Can you work these out from the model? Positions are in its coordinate system, mm. A direction names the side the tool comes from. Give positions to 0.01 mm unless a question says otherwise; leave off trailing zeros. Order: outer loops, then holes, each group sorted by start corner. A loop starts at its lowest first (then second) coordinate and runs counter-clockwise, first axis right, second up.
Item 1: I want a section at C-C, the plane y = 112. Write out the boundary of the cut face in (x, z).
Item 2: Which directions (+Z, -Z, +X, -X, +Y, -Y) give clear straight access to the entire face, cutting with the end or side of a thin tool? Please do faces 4 (the flat face through (-1, 291, -4.034)), 5 (the flat face through (-24.772, 291, 9)).
Item 3: I want a section at A-A, the plane y = 565.15. Write out the boundary of the cut face in (x, z).
Item 4: I'm going to push a flat-ended pin straight in: pin 1 Ø6 at (x, z) = (17, 10) entering from +Y. Where does the tip first touch, or does it pass through?
Item 5: If we mould it in two halves opening along X, with no side actions, what happens to faces 1 (the flat face through (24.504, 291, 9)), 2 (the flat face through (-26.296, 291, 9)), 3 (the flat face through (-1, 291, -2.51))? For each: +X half, -X half, draft (parallel to the pull), parting line (faces both ways), or undercut.
Item 6: I want a section at B-B, the plane z = 11. Write out the boundary of the cut face in (x, y).
Item 7: I want a section at D-D, the plane x = -1. Write out the boundary of the cut face in (y, z).
Item 8: If I drill on line 1 along Z through (x, y) = (-17, 196.5); line 2 along X through (y, z) = (402.5, 8); line 3 along X through (y, z) = (565.15, -3.4), over which ranges is the centre line in solid material (lowest first)?
```python
from build123d import *

# Parameters (mm, degrees)
SKETCH1_W           = 50.8
SKETCH1_H           = 25.4
SKETCH1_W_2         = 47.752
SKETCH1_H_2         = 22.352
BOSS_EXTRUDE2_DEPTH = 590.55
SKETCH2_R           = 7.9375
CUT_EXTRUDE1_DEPTH  = 26.4


with BuildPart() as part:
    # Sketch1 → Boss-Extrude2 (new body)
    with BuildSketch(Plane(origin=(0, 0, 0), x_dir=(1, 0, 0), z_dir=(0, 1, 0))):
        with Locations((-0.896470588, -8.665882353)):
            Rectangle(SKETCH1_W, SKETCH1_H)
        with Locations((-0.896470588, -8.665882353)):
            Rectangle(SKETCH1_W_2, SKETCH1_H_2, mode=Mode.SUBTRACT)
    extrude(amount=BOSS_EXTRUDE2_DEPTH)

    # Sketch2 → Cut-Extrude1 (cut, through all)
    with BuildSketch(Plane.XY.offset(21.365882353)):
        with Locations((-0.896470588, 565.15)):
            Circle(SKETCH2_R)
    extrude(amount=-CUT_EXTRUDE1_DEPTH, mode=Mode.SUBTRACT)


solid = part.part
```
Results list:
1. outline: (-26.3, -4.03) - (24.5, -4.03) - (24.5, 21.37) - (-26.3, 21.37) - close; hole (-24.77, -2.51) - (22.98, -2.51) - (22.98, 19.84) - (-24.77, 19.84) - close
2. face 4: -Z, +X, -X, +Y, -Y
2. face 5: +Y, -Y
3. outline: (-26.3, -4.03) - (-8.83, -4.03) - (-8.83, -2.51) - (-24.77, -2.51) - (-24.77, 19.84) - (-8.83, 19.84) - (-8.83, 21.37) - (-26.3, 21.37) - close; (7.04, -4.03) - (24.5, -4.03) - (24.5, 21.37) - (7.04, 21.37) - (7.04, 19.84) - (22.98, 19.84) - (22.98, -2.51) - (7.04, -2.51) - close
4. pin 1: passes through
5. face 1: +X half
5. face 2: -X half
5. face 3: undercut
6. outline: (-26.3, 0) - (-24.77, 0) - (-24.77, 590.55) - (-26.3, 590.55) - close; (22.98, 0) - (24.5, 0) - (24.5, 590.55) - (22.98, 590.55) - close
7. outline: (0, -4.03) - (557.21, -4.03) - (557.21, -2.51) - (0, -2.51) - close; (0, 19.84) - (557.21, 19.84) - (557.21, 21.37) - (0, 21.37) - close; (573.09, -4.03) - (590.55, -4.03) - (590.55, -2.51) - (573.09, -2.51) - close; (573.09, 19.84) - (590.55, 19.84) - (590.55, 21.37) - (573.09, 21.37) - close
8. line 1: z = -4.03 to -2.51, 19.84 to 21.37
8. line 2: x = -26.3 to -24.77, 22.98 to 24.5
8. line 3: x = -26.3 to -8.83, 7.04 to 24.5
